from build123d import *

# Parameters (mm, degrees)
ESQUISSE1_R             = 5.4
BOSS_EXTRU_1_DEPTH      = 18.3
ESQUISSE2_R             = 7.15
BOSS_EXTRU_3_DEPTH      = 3.4
ESQUISSE3_R             = 4.15
ESQUISSE3_R_2           = 3
ENL_V_MAT_EXTRU_1_DEPTH = 3.4
ESQUISSE5_R             = 2
ENL_V_MAT_EXTRU_2_DEPTH = 3.4
ESQUISSE6_W             = 0.8
ESQUISSE6_H             = 6
BOSS_EXTRU_4_DEPTH      = 8.7


with BuildPart() as part:
    # Esquisse1 → Boss.-Extru.1 (new body)
    with BuildSketch(Plane.XY):
        Circle(ESQUISSE1_R)
    extrude(amount=BOSS_EXTRU_1_DEPTH)

    # Esquisse2 → Boss.-Extru.3 (add)
    with BuildSketch(Plane(origin=(0, 0, 0), x_dir=(-1, 0, 0), z_dir=(0, 0, -1))):
        Circle(ESQUISSE2_R)
    extrude(amount=BOSS_EXTRU_3_DEPTH)

    # Esquisse3 → Enlèv. mat.-Extru.1 (cut)
    with BuildSketch(Plane(origin=(0, 0, -3.4), x_dir=(-1, 0, 0), z_dir=(0, 0, -1))):
        Circle(ESQUISSE3_R)
        Circle(ESQUISSE3_R_2, mode=Mode.SUBTRACT)
    extrude(amount=-ENL_V_MAT_EXTRU_1_DEPTH, mode=Mode.SUBTRACT)

    # Esquisse5 → Enlèv. mat.-Extru.2 (cut)
    with BuildSketch(Plane(origin=(0, 0, -3.4), x_dir=(-1, 0, 0), z_dir=(0, 0, -1))):
        Circle(ESQUISSE5_R)
    extrude(amount=-ENL_V_MAT_EXTRU_2_DEPTH, mode=Mode.SUBTRACT)

    # Esquisse6 → Boss.-Extru.4 (add)
    with BuildSketch(Plane.XY.offset(18.3)):
        Rectangle(ESQUISSE6_W, ESQUISSE6_H)
    extrude(amount=BOSS_EXTRU_4_DEPTH)


solid = part.part
Check sheet for the modelled part. Datum: model origin and axes. Units: mm. A direction names the side the tool comes from. Coordinates: 2 decimals unless noted, no trailing zeros. Write each loop counter-clockwise with the first axis right and the second up, starting at its lowest first coordinate (ties: lowest second). Pieces come first, ordered by that corner, then holes.
Item 1: Cross-section at B-B on x = 0. Record the boundary of the cut face in (y, z).
Numbers:
outline: (-7.15, -3.4) - (-4.15, -3.4) - (-4.15, 0) - (-3, 0) - (-3, -3.4) - (-2, -3.4) - (-2, 0) - (2, 0) - (2, -3.4) - (3, -3.4) - (3, 0) - (4.15, 0) - (4.15, -3.4) - (7.15, -3.4) - (7.15, 0) - (5.4, 0) - (5.4, 18.3) - (3, 18.3) - (3, 27) - (-3, 27) - (-3, 18.3) - (-5.4, 18.3) - (-5.4, 0) - (-7.15, 0) - close
Item 2: Cross-section at A-A on y = 0. Record the boundary of the cut face in (x, z).
Numbers:
outline: (-7.15, -3.4) - (-4.15, -3.4) - (-4.15, 0) - (-3, 0) - (-3, -3.4) - (-2, -3.4) - (-2, 0) - (2, 0) - (2, -3.4) - (3, -3.4) - (3, 0) - (4.15, 0) - (4.15, -3.4) - (7.15, -3.4) - (7.15, 0) - (5.4, 0) - (5.4, 18.3) - (0.4, 18.3) - (0.4, 27) - (-0.4, 27) - (-0.4, 18.3) - (-5.4, 18.3) - (-5.4, 0) - (-7.15, 0) - close
Item 3: Access from +Z, -Z, +X, -X, +Y, -Y to the whole of each face (thin tool, end or side, straight path). Record for faces 5 (the face through (-1, -2, -3.4)), 6 (the face through (-1.17, -5.27, 9.02)), 7 (the face through (0.4, 0, 23)), 8 (the face through (0, -2, -2)), 9 (the face through (0.93, 7.09, -1.68)).
Numbers:
face 5: -Z, +X, -X, +Y, -Y
face 6: +Z
face 7: +Z, +X, +Y, -Y
face 8: -Z
face 9: +Z, -Z
Item 4: Cross-section at C-C on z = 12. Record the boundary of the cut face in (x, y), then the cut area to 3 significant figures.
Numbers:
outline: circle Ø10.8 at (0, 0)
area: 91.6 mm2
Item 5: Scan lines: probe 1 along Y at (x, z) = (0, -1.1); probe 2 along Z at (x, y) = (6.25, 2.5); probe 3 along Z at (x, y) = (2, -4.75). Record each from-to range of solid material in increasing order.
Numbers:
probe 1: y = -7.15 to -4.15, -3 to -2, 2 to 3, 4.15 to 7.15
probe 2: z = -3.4 to 0
probe 3: z = -3.4 to 18.3
Item 6: Depth check by flat-ended pin: pin 1 Ø3 at (y, z) = (-1, 24) entering from +X; pin 2 Ø0.6 at (x, z) = (0, 21.5) entering from +Y; pin 3 Ø6 at (x, z) = (3, 13) entering from +Y. Enter the tip coordinate at first touch or a pass-through.
Numbers:
pin 1: stops at x = 0.4
pin 2: stops at y = 3
pin 3: stops at y = 5.4
Item 7: Cross-section at D-D on y = -5. Record the boundary of the cut face in (x, z), then the cut area to 3 significant figures.
Numbers:
outline: (-5.11, -3.4) - (5.11, -3.4) - (5.11, 0) - (2.04, 0) - (2.04, 18.3) - (-2.04, 18.3) - (-2.04, 0) - (-5.11, 0) - close
area: 109 mm2
Item 8: Mould release check, pull along X, two halves, no side actions. Record for faces 1 (the face through (0.9, -4.05, -1.72)), 2 (the face through (1, 0, 18.3)), 3 (the face through (-0.4, 0, 23)), 4 (the face through (3, 0, -2)): released by +X, released by -X, zero draft, split by the parting line, or undercut.
Numbers:
face 1: undercut
face 2: zero draft
face 3: released by -X
face 4: undercut
